The figure shows three views and two pictorial views of one solid part (mm, origin at its lowest corner). Answer the questions. A direction names the side the tool comes from. Round coordinates to 2 decimals unless told otherwise and drop trailing zeros. Order: outer loops, then holes, each group sorted by start corner. A loop starts at its lowest first (then second) coordinate and runs counter-clockwise, first axis right, second up. Notation, with made-up numbers: (1, 54.5) -> (41, 54.5) arc R16 cw to (41, 70.5) -> close; hole circle Ø8 at (52, 37). An arc over 180 degrees is marked (long way). Answer as a JSON object with one key per item and string values. Group by question number.
Item 1: Given P1, Ø6, axis at x = 2.5, z = 15.5, coming from the +Y side; P2, Ø1.5, axis at x = 3, y = 8.5, coming from the -Z side; P3, Ø2, axis at y = 5, z = 30, coming from the +X side, each flat-ended and moving along its own axis, determine where each tip first touches the part or whether it passes through.
Item 2: For the marked faces 1, 2 and 3, determine the directions among +Z, -Z, +X, -X, +Y, -Y from which every point of the face is accessible in a straight line to the end or side of a thin tool.
Item 3: Section C-C, the plane y = 1.5 is taken. Write down the section's boundary in (x, z), plus the area to 3 significant figures.
Item 4: Section B-B, the plane z = 4 is taken. Write down the section's boundary in (x, y).
Item 5: Section D-D, the plane x = 10.75 is taken. Write down the section's boundary in (y, z).
Item 6: Section A-A, the plane x = 8.75 is taken. Write down the section's boundary in (y, z).
Item 7: Consider probe 1 along Y at (x, z) = (6, 34.35); probe 2 along Z at (x, y) = (7, 11); probe 3 along Y at (x, z) = (9.75, 3). Determine where each line is inside the solid, lowest interval first. Write a range as from..to.
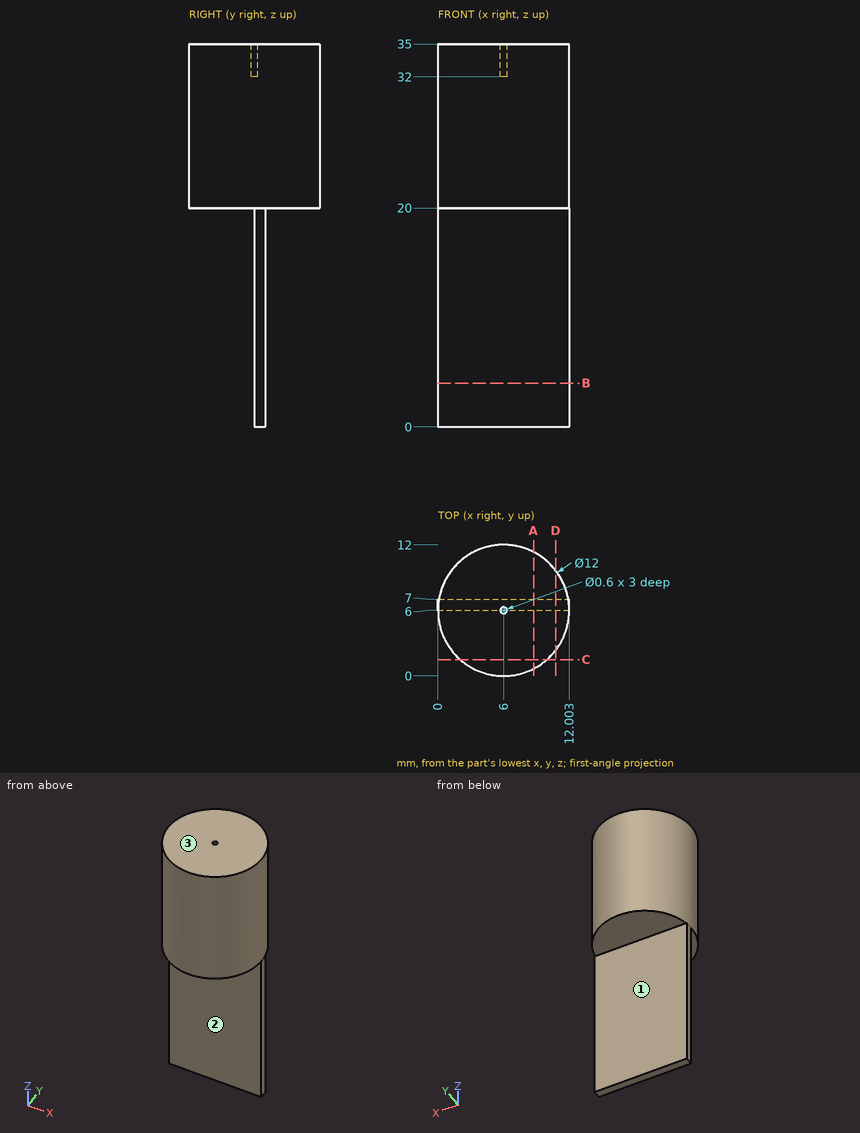
Values found:
{
 "1": {"P1": "y = 7", "P2": "z = 20", "P3": "x = 12"},
 "2": {"face 1": "-Z, +X, -X, +Y", "face 2": "-Z, +X, -X, -Y", "face 3": "+Z, +X, -X, +Y, -Y"},
 "3": {"outline": "(2.03, 20) -> (9.97, 20) -> (9.97, 35) -> (2.03, 35) -> close", "area": "119 mm2"},
 "4": {"outline": "(0, 6) -> (12, 6) -> (12, 7) -> (0, 7) -> close"},
 "5": {"outline": "(2.33, 20) -> (6, 20) -> (6, 0) -> (7, 0) -> (7, 20) -> (9.67, 20) -> (9.67, 35) -> (2.33, 35) -> close"},
 "6": {"outline": "(0.67, 20) -> (6, 20) -> (6, 0) -> (7, 0) -> (7, 20) -> (11.33, 20) -> (11.33, 35) -> (0.67, 35) -> close"},
 "7": {"probe 1": "0..5.7, 6.3..12", "probe 2": "20..35", "probe 3": "6..7"}
}
